Could you check a few things on this model? Use its own coordinates, in mm. Face numbers are marked on the shaded views. A direction names the side the tool comes from. Coordinates: 2 decimals unless noted, no trailing zeros. Loops run counter-clockwise (first coordinate to the right, second up) from the corner with the lowest first, then second, coordinate; pieces in that order, holes last.
1) For the marked faces 3, 4 and 5, which set-ups out of +Z, -Z, +X, -X, +Y, -Y let a thin tool reach every point of the face, with its end or its side?
2) Imagine slicing it at B-B on x = -5.5. Please give me the cut outline in (y, z) (3 decimals).
3) Imagine slicing it at A-A on y = 5. Please give me the cut outline in (x, z) (3 decimals), plus the area to 3 significant figures.
4) Thinking about a two-plate mould opening in Y: for the marked faces 1 and 2, which applies, released by +Y, released by -Y, zero draft, split by the parting line, or undercut?
5) Will these pins go through, and if not, where does the flat tip stop? P1, Ø2, axis at y = 2, z = 8, coming from the +X side; P2, Ø4, axis at y = 2, z = 5, coming from the +X side (3 decimals); P3, Ø1, axis at y = -9.5, z = 8, coming from the -X side; P4, Ø1.5, axis at x = 0, z = 5.5, coming from the +Y side.
6) If I drill on line 1 along X through (y, z) = (6.5, 5.75); line 2 along X through (y, z) = (12, 3); line 3 along Y through (x, z) = (1.5, 1), over which ranges is the centre line in solid material (lowest first)?
7) Imagine slicing it at D-D on x = 0. Please give me the cut outline in (y, z) (3 decimals), plus the area to 3 significant figures.
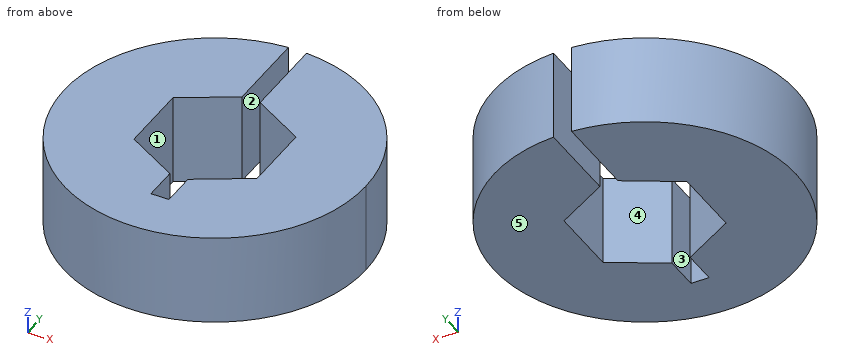
Autodesk Inventor part; units mm, degrees
ref_plane "YZ Plane" through (0, 0, 0) normal (1, 0, 0) x (0, 1, 0)
ref_plane "XZ Plane" through (0, 0, 0) normal (0, 1, 0) x (-1, 0, 0)
ref_plane "XY Plane" through (0, 0, 0) normal (0, 0, 1) x (1, 0, 0)
sketch "Sketch1" plane through (0, 0, 0) normal (0, 0, 1) x (1, 0, 0)
  circle A0 centre (0, 0) radius 15.875
  dimension "d0" = 31.75
extrude "Extrusion1" add sketch "Sketch1" along normal blind 9.525
sketch "Sketch2" plane through (0, 0, 9.525) normal (0, 0, 1) x (1, 0, 0)
  line L0 (-6.477, -3.7395) -> (-6.477, 3.7395)
  line L1 (-6.477, 3.7395) -> (0, 7.479)
  line L2 (0, 7.479) -> (6.477, 3.7395)
  line L3 (6.477, 3.7395) -> (6.477, -3.7395)
  line L4 (6.477, -3.7395) -> (0, -7.479)
  line L5 (0, -7.479) -> (-6.477, -3.7395)
  circle A0 centre (0, 0) radius 15.875
  line L6 (-0.9525, 15.8464) -> (-0.9525, -10.5696)
  line L7 (-0.9525, -10.5696) -> (0.9525, -10.5696)
  line L8 (0.9525, -10.5696) -> (0.9525, 15.8464)
  arc A1 (0.9525, 15.8464) -> (-0.9525, 15.8464) centre (0, 0) ccw
  point P0 (-6.477, 0)
  dimension "d3" = 12.954
  dimension "d4" = 1.905
  dimension "d5" = 0.9525
  dimension "d6" = 26.416
extrude "Extrusion2" cut sketch "Sketch2" against normal blind 9.525 contours L0 L1 L6 L5 | L6 L1 L2 L8 L4 L5 | L5 L4 L8 L7 L6 | L6 A0 L8 L2 L1 | L8 L2 L3 L4
equation "\"d5\" = 0.5 * d4"
properties part number "Collar"
Filled in:
1. face 3: +Z, -Z, +Y
1. face 4: +Z, -Z
1. face 5: -Z, +X, -X, +Y, -Y
2. outline: (-14.892, 0) - (-4.304, 0) - (-4.304, 9.525) - (-14.892, 9.525) - close; (4.304, 0) - (14.892, 0) - (14.892, 9.525) - (4.304, 9.525) - close
3. outline: (-15.067, 0) - (-4.294, 0) - (-4.294, 9.525) - (-15.067, 9.525) - close; (4.294, 0) - (15.067, 0) - (15.067, 9.525) - (4.294, 9.525) - close
3. area: 205 mm2
4. face 1: undercut
4. face 2: zero draft
5. P1: stops at x = 15.84
5. P2: stops at x = 15.875
5. P3: stops at x = -13.08
5. P4: stops at y = -10.57
6. line 1: x = -14.48 to -1.7, 1.7 to 14.48
6. line 2: x = -10.39 to -0.95, 0.95 to 10.39
6. line 3: y = -15.8 to -6.61, 6.61 to 15.8
7. outline: (-15.875, 0) - (-10.57, 0) - (-10.57, 9.525) - (-15.875, 9.525) - close
7. area: 50.5 mm2
